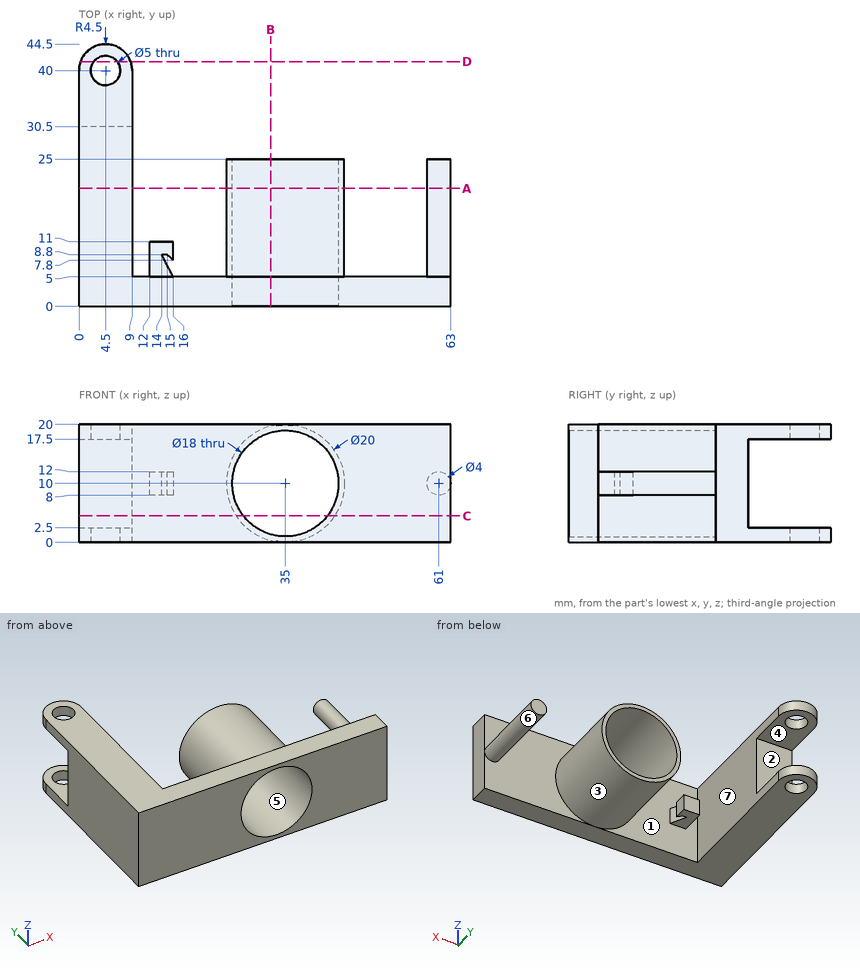
Print and shaded views of the part. All mm, measured from the part's lowest x, y and z. A direction names the side the tool comes from. Coordinates: 2 decimals unless noted, no trailing zeros. Order: outer loops, then holes, each group sorted by start corner. A loop starts at its lowest first (then second) coordinate and runs counter-clockwise, first axis right, second up.
(1) Pull direction Z, two halves, no side cores. Call the marked faces 1, 2, 3 and 4: pulls with the +Z half, pulls with the -Z half, needs draft (parallel to the pull), parting line crosses it, or undercut.
Check sheet entries:
face 1: needs draft
face 2: undercut
face 3: parting line crosses it
face 4: undercut
(2) Slice it at D-D, the plane y = 41.5. Write the cut outline in (x, z).
Check sheet entries:
outline: (0.26, 0) - (2.5, 0) - (2.5, 2.5) - (0.26, 2.5) - close; (0.26, 17.5) - (2.5, 17.5) - (2.5, 20) - (0.26, 20) - close; (6.5, 0) - (8.74, 0) - (8.74, 2.5) - (6.5, 2.5) - close; (6.5, 17.5) - (8.74, 17.5) - (8.74, 20) - (6.5, 20) - close
(3) Probe L1, parallel to X at y = 40, z = 18.4; L2, parallel to Y at x = 4.5, z = 0.75; L3, parallel to X at y = 6.5, z = 10. List the from-to ranges inside material, lowest first.
Check sheet entries:
L1: x = 0 to 2, 7 to 9
L2: y = 0 to 37.5, 42.5 to 44.5
L3: x = 0 to 9, 12 to 15.21, 25 to 26, 44 to 45, 59 to 63
(4) Slice it at B-B, the plane x = 32.5. Write the cut outline in (y, z), and give its area (3 significant figures).
Check sheet entries:
outline: (0, 0) - (5, 0) - (5, 0.32) - (25, 0.32) - (25, 1.35) - (0, 1.35) - close; (0, 18.65) - (25, 18.65) - (25, 19.68) - (5, 19.68) - (5, 20) - (0, 20) - close
area: 55.0 mm2
(5) Slice it at C-C, the plane z = 4.5. Write the cut outline in (x, y), and give its area (3 significant figures).
Check sheet entries:
outline: (0, 0) - (27.88, 0) - (27.88, 25) - (26.65, 25) - (26.65, 5) - (9, 5) - (9, 30.5) - (0, 30.5) - close; (42.12, 0) - (63, 0) - (63, 5) - (43.35, 5) - (43.35, 25) - (42.12, 25) - close
area: 522 mm2
(6) Tool access for the marked faces 5, 6 and 7: list every direction of +Z, -Z, +X, -X, +Y, -Y with a clear straight run to the whole face (end or side of a thin tool).
Check sheet entries:
face 5: +Y, -Y
face 6: +Y
face 7: +Z, -Z, +Y
(7) Slice it at A-A, the plane y = 20. Write the cut outline in (x, z).
Check sheet entries:
outline: (0, 0) - (9, 0) - (9, 20) - (0, 20) - close; circle Ø20 at (35, 10); circle Ø4 at (61, 10); hole circle Ø18 at (35, 10)
(8) Pin check, flat tips, straight feed: pin 1 Ø3 at (x, y) = (4.5, 40) entering from +Z; pin 2 Ø8 at (x, y) = (10.5, 32.5) entering from -Z; pin 3 Ø6 at (x, y) = (28.5, 21.5) entering from +Z; pin 4 Ø1 at (x, y) = (38, 12) entering from -Z. Stop position of each tip, or through.
Check sheet entries:
pin 1: passes through
pin 2: stops at z = 0
pin 3: stops at z = 19.37
pin 4: stops at z = 0.32
